Source: CAD feature listing. Evaluate the final solid. Frame: model axes, mm. A direction names the side the tool comes from. Give positions to 0.01 mm unless a question says otherwise; leave off trailing zeros. Loops run counter-clockwise (first coordinate to the right, second up) from the corner with the lowest first, then second, coordinate; pieces in that order, holes last. Notation, with made-up numbers: M 50,55.5 L 67,55.5 A16 cw 67,73.5 Z; hole C 42,89.25 d5. An arc over 180 degrees is marked long. Answer in a Markdown table with one row per item.
```python
from build123d import *

# Parameters (mm, degrees)
SKETCH1_R               = 1.7
SKETCH1_W               = 6
SKETCH1_H               = 5.5
BOSS_EXTRUDE1_DEPTH     = 3
CUT_EXTRUDE1_DEPTH      = 13.389511693
CUT_EXTRUDE1_DEPTH_BACK = 13.389511693
SKETCH2_W               = 6.1
SKETCH2_H               = 0.75
FILLET2_R               = 1
FILLET1_R               = 1


with BuildPart() as part:
    # Sketch1 → Boss-Extrude1 (new body)
    # profile 1 of 2: a face of its own
    with BuildSketch(Plane.XY):
        with BuildLine():
            Line((-5.5, 3), (5.5, 3))
            ThreePointArc((5.5, 3), (8.5, 0), (5.5, -3))
            Line((5.5, -3), (-5.5, -3))
            ThreePointArc((-5.5, -3), (-8.5, 0), (-5.5, 3))
        make_face()
        with Locations((5.5, 0)):
            Circle(SKETCH1_R, mode=Mode.SUBTRACT)
        with Locations((-5.5, 0)):
            Circle(SKETCH1_R, mode=Mode.SUBTRACT)
    # profile 2 of 2: a face of its own
    with BuildSketch(Plane.XY):
        with Locations((0, 5.75)):
            Rectangle(SKETCH1_W, SKETCH1_H)
    extrude(amount=BOSS_EXTRUDE1_DEPTH)

    # Sketch2 → Cut-Extrude1 (cut, two sides: drawn at the far end of the back side and taken through both)
    with BuildSketch(Plane(origin=(0, 0, 0), x_dir=(1, 0, 0), z_dir=(0, 1, 0)).offset(-CUT_EXTRUDE1_DEPTH_BACK)):
        with Locations((0, -0.375)):
            Rectangle(SKETCH2_W, SKETCH2_H)
    extrude(amount=CUT_EXTRUDE1_DEPTH + CUT_EXTRUDE1_DEPTH_BACK, mode=Mode.SUBTRACT)

    # Fillet2
    fillet2_edges = [part.edges().sort_by_distance(p)[0] for p in [
        (3, 3, 1.875),
        (-3, 3, 1.875),
        (3, 8.5, 1.875),
        (-3, 8.5, 1.875),
    ]]
    fillet(fillet2_edges, radius=FILLET2_R)

    # Fillet1
    # the kernel refuses this fillet: 1 mm, written as the material it takes off along each edge
    with BuildSketch(Plane(origin=(-5.5, 0, 3), x_dir=(0, -1, 0), z_dir=(1, 0, 0))) as fillet1_piece_1:
        with BuildLine():
            CenterArc((3 - FILLET1_R, FILLET1_R), FILLET1_R, 270, 90)
            Line((3, FILLET1_R), (3, 0))
            Line((3, 0), (3 - FILLET1_R, 0))
        make_face()
    revolve(axis=Axis((-5.5, 0, 3), (0, 0, -1)), revolution_arc=180, mode=Mode.SUBTRACT)
    with BuildSketch(Plane(origin=(5.5, -3, 3), x_dir=(0, 0, -1), z_dir=(-1, 0, 0))) as fillet1_piece_2:
        with BuildLine():
            CenterArc((FILLET1_R, -FILLET1_R), FILLET1_R, 90, 90)
            Line((0, -FILLET1_R), (0, 0))
            Line((0, 0), (FILLET1_R, 0))
        make_face()
    extrude(amount=11, mode=Mode.SUBTRACT)
    with BuildSketch(Plane(origin=(5.5, 0, 3), x_dir=(0, 1, 0), z_dir=(-1, 0, 0))) as fillet1_piece_3:
        with BuildLine():
            CenterArc((3 - FILLET1_R, FILLET1_R), FILLET1_R, 270, 90)
            Line((3 - FILLET1_R, 0), (3, 0))
            Line((3, 0), (3, FILLET1_R))
        make_face()
    revolve(axis=Axis((5.5, 0, 3), (0, 0, -1)), revolution_arc=180, mode=Mode.SUBTRACT)
    with BuildSketch(Plane(origin=(3.05, -3, -2.5), x_dir=(0, 1, 0), z_dir=(0, 0, 1))) as fillet1_piece_4:
        with BuildLine():
            CenterArc((FILLET1_R, -FILLET1_R), FILLET1_R, 90, 90)
            Line((0, -FILLET1_R), (0, 0))
            Line((0, 0), (FILLET1_R, 0))
        make_face()
    extrude(amount=3.25, mode=Mode.SUBTRACT)
    with BuildSketch(Plane(origin=(-3.05, -3, 0.75), x_dir=(-1, 0, 0), z_dir=(0, 0, -1))) as fillet1_piece_5:
        with BuildLine():
            CenterArc((FILLET1_R, FILLET1_R), FILLET1_R, 180, 90)
            Line((0, FILLET1_R), (0, 0))
            Line((0, 0), (FILLET1_R, 0))
        make_face()
    extrude(amount=3.25, mode=Mode.SUBTRACT)
    with BuildSketch(Plane(origin=(-5.5, 3, 3), x_dir=(0, -1, 0), z_dir=(1, 0, 0))) as fillet1_piece_6:
        with BuildLine():
            CenterArc((FILLET1_R, FILLET1_R), FILLET1_R, 180, 90)
            Line((0, FILLET1_R), (0, 0))
            Line((0, 0), (FILLET1_R, 0))
        make_face()
    extrude(amount=1.5, mode=Mode.SUBTRACT)
    with BuildSketch(Plane(origin=(4, 3, 3), x_dir=(0, 0, -1), z_dir=(1, 0, 0))) as fillet1_piece_7:
        with BuildLine():
            CenterArc((FILLET1_R, -FILLET1_R), FILLET1_R, 90, 90)
            Line((0, -FILLET1_R), (0, 0))
            Line((0, 0), (FILLET1_R, 0))
        make_face()
    extrude(amount=1.5, mode=Mode.SUBTRACT)
    with BuildSketch(Plane(origin=(4, 4, 3), x_dir=(0, -1, 0), z_dir=(1, 0, 0))) as fillet1_piece_8:
        with BuildLine():
            CenterArc((1 + FILLET1_R, FILLET1_R), FILLET1_R, 180, 90)
            Line((1 + FILLET1_R, 0), (1, 0))
            Line((1, 0), (1, FILLET1_R))
        make_face()
    revolve(axis=Axis((4, 4, 3), (0, 0, -1)), revolution_arc=90, mode=Mode.SUBTRACT)
    with BuildSketch(Plane(origin=(3, 4, 3), x_dir=(-1, 0, 0), z_dir=(0, 1, 0)), Plane(origin=(-3, 7.5, 3), x_dir=(1, 0, 0), z_dir=(0, -1, 0))) as fillet1_piece_9:
        with BuildLine():
            CenterArc((FILLET1_R, -FILLET1_R), FILLET1_R, 90, 90)
            Line((0, -FILLET1_R), (0, 0))
            Line((0, 0), (FILLET1_R, 0))
        make_face()
    extrude(amount=3.5, mode=Mode.SUBTRACT)
    with BuildSketch(Plane(origin=(2, 7.5, 3), x_dir=(0, 1, 0), z_dir=(-1, 0, 0))) as fillet1_piece_10:
        with BuildLine():
            CenterArc((1 - FILLET1_R, FILLET1_R), FILLET1_R, 270, 90)
            Line((1, FILLET1_R), (1, 0))
            Line((1, 0), (1 - FILLET1_R, 0))
        make_face()
    revolve(axis=Axis((2, 7.5, 3), (0, 0, -1)), revolution_arc=90, mode=Mode.SUBTRACT)
    with BuildSketch(Plane(origin=(2, 8.5, 3), x_dir=(0, -1, 0), z_dir=(-1, 0, 0))) as fillet1_piece_11:
        with BuildLine():
            CenterArc((FILLET1_R, -FILLET1_R), FILLET1_R, 90, 90)
            Line((0, -FILLET1_R), (0, 0))
            Line((0, 0), (FILLET1_R, 0))
        make_face()
    extrude(amount=4, mode=Mode.SUBTRACT)
    with BuildSketch(Plane(origin=(-2, 7.5, 3), x_dir=(-1, 0, 0), z_dir=(0, -1, 0))) as fillet1_piece_12:
        with BuildLine():
            CenterArc((1 - FILLET1_R, FILLET1_R), FILLET1_R, 270, 90)
            Line((1, FILLET1_R), (1, 0))
            Line((1, 0), (1 - FILLET1_R, 0))
        make_face()
    revolve(axis=Axis((-2, 7.5, 3), (0, 0, -1)), revolution_arc=90, mode=Mode.SUBTRACT)
    with BuildSketch(Plane(origin=(-4, 4, 3), x_dir=(0, -1, 0), z_dir=(-1, 0, 0))) as fillet1_piece_13:
        with BuildLine():
            CenterArc((1 + FILLET1_R, -FILLET1_R), FILLET1_R, 90, 90)
            Line((1, -FILLET1_R), (1, 0))
            Line((1, 0), (1 + FILLET1_R, 0))
        make_face()
    revolve(axis=Axis((-4, 4, 3), (0, 0, 1)), revolution_arc=90, mode=Mode.SUBTRACT)
    with BuildSketch(Plane(origin=(-3.05, 3.6877501, -4.21937525), x_dir=(0, -1, 0), z_dir=(0, 0, 1))) as fillet1_piece_14:
        with BuildLine():
            CenterArc((1.6877501, -1), FILLET1_R, 90, 90)
            Line((0.6877501, -1), (0.5877501, -1))
            ThreePointArc((0.5877501, -1), (0.5877501, -0.95), (-0.03122499, -0.095))
            Line((-0.03122499, -0.095), (0, 0.1))
            Line((0, 0.1), (1.6877501, 0.1))
            Line((1.6877501, 0.1), (1.6877501, 0))
        make_face()
    extrude(amount=4.96937525, mode=Mode.SUBTRACT)
    with BuildSketch(Plane(origin=(3.05, 3.6877501, -4.21937525), x_dir=(0.8239457103973873, -0.5666687447863566, 0), z_dir=(0, 0, 1))) as fillet1_piece_15:
        with BuildLine():
            CenterArc((1.780340941, -0.82394571), FILLET1_R, 124.51825235, 90)
            Line((0.956395231, -1.390614455), (0.87400066, -1.44728133))
            Line((0.87400066, -1.44728133), (-0.082394571, -0.056666874))
            Line((-0.082394571, -0.056666874), (0.060580617, 0.079561227))
            ThreePointArc((0.060580617, 0.079561227), (1.115808036, 0.054061134), (1.157005322, 0.082394571))
            Line((1.157005322, 0.082394571), (1.213672196, 0))
        make_face()
    extrude(amount=4.96937525, mode=Mode.SUBTRACT)


solid = part.part
```
1) Material intervals for L1, parallel to Y at x = 5.5, z = 1.3; L2, parallel to X at y = 1.5, z = 2.6; L3, parallel to X at y = 5.5, z = 1.6, sorted ascending.
Reply:
| item | result |
|---|---|
| L1 | y = -3 to -1.7, 1.7 to 3 |
| L2 | x = -7.86 to -6.3, -4.7 to 4.7, 6.3 to 7.86 |
| L3 | x = -3 to 3 |
2) Section C-C, the plane x = 4.5. Return loops of the section in (y, z).
Reply:
| item | result |
|---|---|
| outline | M -3,0 L -1.37,0 L -1.37,3 L -2,3 A1 ccw -3,2 Z; M 1.37,0 L 3,0 L 3,2 A1 ccw 2,3 L 1.37,3 Z |
3) Pin query (flat end, axial travel): pin 1 Ø4 at (x, y) = (2, 3) entering from -Z; pin 2 Ø0.6 at (y, z) = (5.5, 1.5) entering from +X; pin 3 Ø0.6 at (y, z) = (0.5, 0.5) entering from -X; pin 4 Ø1 at (y, z) = (6.5, 1.5) entering from -X. Return the tip coordinate at first contact, or that it passes through.
Reply:
| item | result |
|---|---|
| pin 1 | stops at z = 0 |
| pin 2 | stops at x = 3 |
| pin 3 | stops at x = -8.49 |
| pin 4 | stops at x = -3 |
4) Section A-A, the plane y = 0. Return loops of the section in (x, z), then the cut area to 3 significant figures.
Reply:
| item | result |
|---|---|
| outline | M -8.5,0 L -7.2,0 L -7.2,3 L -7.5,3 A1 ccw -8.5,2 Z; M -3.8,0 L -3.05,0 L -3.05,0.75 L 3.05,0.75 L 3.05,0 L 3.8,0 L 3.8,3 L -3.8,3 Z; M 7.2,0 L 8.5,0 L 8.5,2 A1 ccw 7.5,3 L 7.2,3 Z |
| area | 25.6 mm² |
5) Pull-direction query (X, two-part tool) for faces 1 (the cylindrical face through (-3.335, 2.699, 0.37)), 2 (the flat face through (0, -3, 1)), 3 (the flat face through (-3, 6, 1)); classes: released by +X, released by -X, zero draft, split by the parting line, or undercut.
Reply:
| item | result |
|---|---|
| face 1 | undercut |
| face 2 | zero draft |
| face 3 | released by -X |
6) Section D-D, the plane y = 6.5. Return loops of the section in (x, z).
Reply:
| item | result |
|---|---|
| outline | M -3,0.75 L 3,0.75 L 3,2 A1 ccw 2,3 L -2,3 A1 ccw -3,2 Z |
7) Section B-B, the plane z = 1.8. Return loops of the section in (x, y).
Reply:
| item | result |
|---|---|
| outline | M -5.5,-3 L 5.5,-3 A3 ccw 5.5,3 L 4,3 A1 cw 3,4 L 3,7.5 A1 ccw 2,8.5 L -2,8.5 A1 ccw -3,7.5 L -3,4 A1 cw -4,3 L -5.5,3 A3 ccw Z; hole C -5.5,0 d3.4; hole C 5.5,0 d3.4 |
8) Set-up query: faces 4 (the cylindrical face through (-3.335, -2.699, 0.38)), 5 (the flat face through (-5, 3, 1)), 6 (the flat face through (3, 6, 1)). Return all of +Z, -Z, +X, -X, +Y, -Y with unobstructed straight access to the full face (end or side cutting, diameter ignored); none if empty.
Reply:
| item | result |
|---|---|
| face 4 | -Z, -Y |
| face 5 | +Z, -Z, -X, +Y |
| face 6 | +Z, -Z, +X, +Y |
